Work out the finished part from the listing and answer in its coordinate system (mm). A direction names the side the tool comes from. Round coordinates to 2 decimals unless told otherwise and drop trailing zeros. Write each loop counter-clockwise with the first axis right and the second up, starting at its lowest first coordinate (ties: lowest second). Pieces come first, ordered by that corner, then holes. Notation, with made-up numbers: M 46,24.5 L 85,24.5 A11 cw 85,31.5 Z; hole C 56.5,59 d9. An arc over 180 degrees is marked long. One line per item, written item: value. Start each with the question number.
Q1. Find section A-A (x = 0). Write down the section's boundary in (y, z), and give its area (3 significant figures).
Q2. Find section C-C (z = 13.75). Write down the section's boundary in (x, y), and give its area (3 significant figures).
Q3. Given pin 1 Ø1.5 at (x, y) = (0, 3) entering from +Z; pin 2 Ø2 at (y, z) = (-7, 8) entering from -X; pin 3 Ø6 at (x, z) = (5.5, 15.5) entering from +Y, each flat-ended and moving along its own axis, determine where each tip first touches the part or whether it passes through.
Q4. A tool of negligible diameter and unlimited length cuts with its end or side. For faces 1 (the flat face through (0, 0, 0)), 2 (the flat face through (0, 0, 6.35)), from which of +Z, -Z, +X, -X, +Y, -Y can it reach the whole face along a straight path? Write none if from no direction.
Q5. Consider probe 1 along Y at (x, z) = (0, 10.25); probe 2 along Z at (x, y) = (-4, -1); probe 3 along Y at (x, z) = (-5, 22.75). Determine where each line is inside the solid, lowest interval first.
Q6. The mould has two halves that part along X. Classify faces 3 (the flat face through (-2, -7, 25.4)), 4 (the cylindrical face through (-1.34, -6.01, 15.62)), 5 (the cylindrical face through (-2.12, -9.546, 12.533)): released by +X, released by -X, zero draft, split by the parting line, or undercut.
from build123d import *

# Parameters (mm, degrees)
F0_R     = 9.779
F1_DEPTH = 25.4
F2_SIZE  = 0.762
F3_R     = 6.1595
F4_DEPTH = 19.05
F5_SIZE  = 0.762


with BuildPart() as f1:
    # F0 (on Top) → F1 (new body)
    with BuildSketch(Plane.XY):
        Circle(F0_R)
    extrude(amount=F1_DEPTH)

    # F2
    f2_edges = [f1.edges().sort_by_distance(p)[0] for p in [
        (-9.779, 0, 0),
    ]]
    chamfer(f2_edges, length=F2_SIZE)

    # F3 (on face) → F4 (cut)
    with BuildSketch(Plane.XY.offset(25.4)):
        Circle(F3_R)
    extrude(amount=-F4_DEPTH, mode=Mode.SUBTRACT)

    # F5
    f5_edges = [f1.edges().sort_by_distance(p)[0] for p in [
        (-9.779, 0, 25.4),
        (-6.1595, 0, 25.4),
    ]]
    chamfer(f5_edges, length=F5_SIZE)


solid = f1.part
The answers:
1. outline: M -9.78,0.76 L -9.02,0 L 9.02,0 L 9.78,0.76 L 9.78,24.64 L 9.02,25.4 L 6.92,25.4 L 6.16,24.64 L 6.16,6.35 L -6.16,6.35 L -6.16,24.64 L -6.92,25.4 L -9.02,25.4 L -9.78,24.64 Z
1. area: 260 mm2
2. outline: C 0,0 d19.56; hole C 0,0 d12.32
2. area: 181 mm2
3. pin 1: z = 6.35
3. pin 2: x = -7.72
3. pin 3: y = 9.45
4. face 1: -Z, +X, -X, +Y, -Y
4. face 2: +Z
5. probe 1: -9.78 to -6.16, 6.16 to 9.78
5. probe 2: 0 to 6.35
5. probe 3: -8.4 to -3.6, 3.6 to 8.4
6. face 3: zero draft
6. face 4: undercut
6. face 5: split by the parting line
